For this review, take the finished solid that the model builds, in its own axes (mm). Coordinates: 2 decimals unless noted, no trailing zeros. Order: outer loops, then holes, each group sorted by start corner. A loop starts at its lowest first (then second) coordinate and runs counter-clockwise, first axis right, second up.
from build123d import *

# Parameters (mm, degrees)
F0_R     = 3.302
F0_R_2   = 10.795
F1_DEPTH = 3.175


with BuildPart() as f1:
    # F0 (on Front) → F1 (new body)
    with BuildSketch(Plane.XZ):
        Polygon((42.291, -24.41672), (0, 48.83344), (-42.291, -24.41672), align=None)
        with Locations((-27.496307, -15.875)):
            Circle(F0_R, mode=Mode.SUBTRACT)
        with Locations((27.496307, -15.875)):
            Circle(F0_R, mode=Mode.SUBTRACT)
        Circle(F0_R_2, mode=Mode.SUBTRACT)
        with Locations((0, 31.75)):
            Circle(F0_R, mode=Mode.SUBTRACT)
    extrude(amount=F1_DEPTH)


solid = f1.part
1. Take a section at B-B, the plane y = -1.4. Give the boundary of the cut face in (x, z) (3 decimals), plus the area to 3 significant figures.
Answer below:
outline: (-42.291, -24.417) - (42.291, -24.417) - (0, 48.833) - close; hole circle Ø6.604 at (-27.496, -15.875); hole circle Ø21.59 at (0, 0); hole circle Ø6.604 at (0, 31.75); hole circle Ø6.604 at (27.496, -15.875)
area: 2,630 mm2
2. Clearance check with a flat-ended pin moving along its axis: pin 1 Ø6 at (x, z) = (27.5, -15.88) entering from +Y. State where the tip first meets the part, or that it passes through.
Answer below:
pin 1: passes through
3. The part is to be moulded in two halves that separate along Z. For faces 1 (the face through (30.547, -1.565, -17.14)), 2 (the face through (21.44, -1.57, 11.7)), 3 (the face through (-10, 0, 5)), say which applies: +Z half, -Z half, draft (parallel to the pull), parting line (faces both ways), or undercut.
Answer below:
face 1: undercut
face 2: +Z half
face 3: draft
4. Take a section at C-C, the plane x = -27. Give the boundary of the cut face in (y, z) (3 decimals), plus the area to 3 significant figures.
Answer below:
outline: (-3.175, -24.417) - (0, -24.417) - (0, -19.139) - (-3.175, -19.139) - close; (-3.175, -12.611) - (0, -12.611) - (0, 2.068) - (-3.175, 2.068) - close
area: 63.4 mm2
5. Take a section at D-D, the plane x = 16. Give the boundary of the cut face in (y, z) (3 decimals), plus the area to 3 significant figures.
Answer below:
outline: (-3.175, -24.417) - (0, -24.417) - (0, 21.121) - (-3.175, 21.121) - close
area: 145 mm2
6. To check wall thickness, follow L1, parallel to X at y = -1.7, z = -13.5; L2, parallel to Z at x = 4.5, y = -2.85; L3, parallel to X at y = -1.6, z = -2. State the ranges of each line that lie inside material, in increasing order.
Answer below:
L1: x = -35.99 to -29.79, -25.2 to 25.2, 29.79 to 35.99
L2: z = -24.42 to -9.81, 9.81 to 41.04
L3: x = -29.35 to -10.61, 10.61 to 29.35
7. Take a section at A-A, the plane z = 2.5. Give the boundary of the cut face in (x, y) (3 decimals), plus the area to 3 significant figures.
Answer below:
outline: (-26.751, -3.175) - (-10.502, -3.175) - (-10.502, 0) - (-26.751, 0) - close; (10.502, -3.175) - (26.751, -3.175) - (26.751, 0) - (10.502, 0) - close
area: 103 mm2
